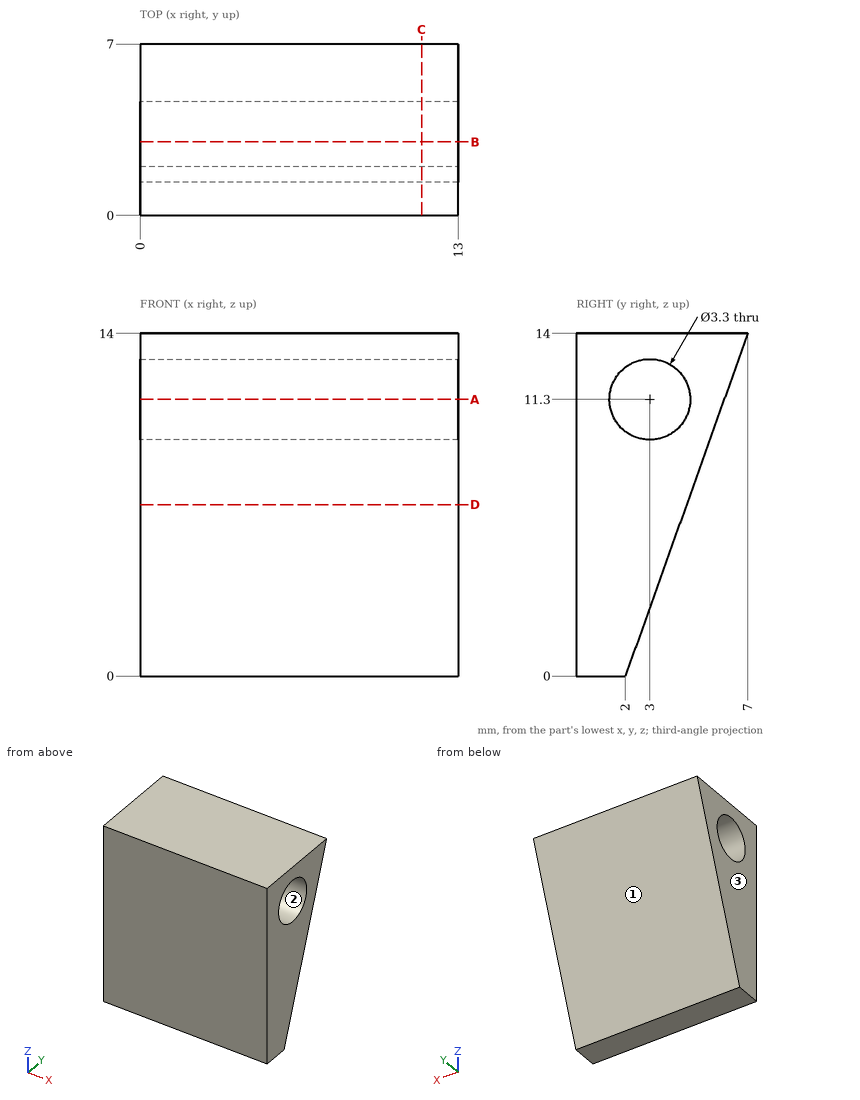
Input: dimensioned drawing with shaded views. Units: mm. Origin: part minimum x, y, z. Give positions to 0.01 mm unless a question says otherwise; leave off trailing zeros. Write each loop counter-clockwise with the first axis right and the second up, starting at its lowest first coordinate (ties: lowest second). Pieces come first, ordered by that corner, then holes. Notation, with made-up numbers: (72.5, -17) - (89.5, -17) arc R24 ccw to (89.5, -2) - close; hole circle Ø2 at (19, 59). An arc over 180 degrees is marked (long way). One line per item, written item: value. Start each with the question number.
Q1. Section query D-D, the plane z = 7. Return the cut outline in (x, y).
Q2. Section query B-B, the plane y = 3. Return the cut outline in (x, z).
Q3. Section query C-C, the plane x = 11.5. Return the cut outline in (y, z).
Q4. Section query A-A, the plane z = 11.3. Return the cut outline in (x, y), then the cut area to 3 significant figures.
Q5. Draft query along Y for the marked faces 1, 2 and 3. Return one class per face: +Y half, -Y half, draft (parallel to the pull), parting line (faces both ways), or undercut.
Q6. Material intervals for probe 1 along Y at (x, z) = (9.75, 11.3); probe 2 along Y at (x, z) = (4.5, 11.75); probe 3 along Z at (x, y) = (5.5, 1.75), sorted ascending. Write a range as from..to.
Q7. First-contact query: pin 1 Ø5 at (x, z) = (10.5, 9) entering from +Y. Flat tip, straight axial feed; report the tip coordinate or a pass-through.
Answer:
1. outline: (0, 0) - (13, 0) - (13, 4.5) - (0, 4.5) - close
2. outline: (0, 2.8) - (13, 2.8) - (13, 9.65) - (0, 9.65) - close; (0, 12.95) - (13, 12.95) - (13, 14) - (0, 14) - close
3. outline: (0, 0) - (2, 0) - (7, 14) - (0, 14) - close; hole circle Ø3.3 at (3, 11.3)
4. outline: (0, 0) - (13, 0) - (13, 1.35) - (0, 1.35) - close; (0, 4.65) - (13, 4.65) - (13, 6.04) - (0, 6.04) - close
4. area: 35.6 mm2
5. face 1: +Y half
5. face 2: undercut
5. face 3: draft
6. probe 1: y = 0..1.35, 4.65..6.04
6. probe 2: y = 0..1.41, 4.59..6.2
6. probe 3: z = 0..10.22, 12.38..14
7. pin 1: stops at y = 6.11
